```python
from build123d import *

# Parameters (mm, degrees)
BOSS_EXTRU_1_DEPTH      = 3.5
ENL_V_MAT_EXTRU_1_DEPTH = 0.2
ESQUISSE3_R             = 2.3
BOSS_EXTRU_2_DEPTH      = 1.3
CONG_1_R                = 0.1
CONG_2_R                = 0.01
ESQUISSE4_W             = 1.998545811
ESQUISSE4_H             = 1.004796591
BOSS_EXTRU_3_DEPTH      = 0.1
ESQUISSE5_W             = 2.001116517
ESQUISSE5_H             = 1.004085413
BOSS_EXTRU_4_DEPTH      = 0.1


with BuildPart() as part:
    # Esquisse1 → Boss.-Extru.1 (new body)
    with BuildSketch(Plane.XY):
        with BuildLine():
            Line((0.5, 0), (5.5, 0))
            ThreePointArc((5.5, 0), (5.853553391, 0.146446609), (6, 0.5))
            Line((6, 0.5), (6, 5.5))
            ThreePointArc((6, 5.5), (5.853553391, 5.853553391), (5.5, 6))
            Line((5.5, 6), (0.5, 6))
            ThreePointArc((0.5, 6), (0.146446609, 5.853553391), (0, 5.5))
            Line((0, 5.5), (0, 0.5))
            ThreePointArc((0, 0.5), (0.146446609, 0.146446609), (0.5, 0))
        make_face()
    extrude(amount=BOSS_EXTRU_1_DEPTH)

    # Esquisse2 → Enlèv. mat.-Extru.1 (cut)
    with BuildSketch(Plane.XY.offset(3.5)):
        with BuildLine():
            Line((1.11, 0.61), (4.89, 0.61))
            ThreePointArc((4.89, 0.61), (5.243553391, 0.756446609), (5.39, 1.11))
            Line((5.39, 1.11), (5.39, 4.89))
            ThreePointArc((5.39, 4.89), (5.243553391, 5.243553391), (4.89, 5.39))
            Line((4.89, 5.39), (1.11, 5.39))
            ThreePointArc((1.11, 5.39), (0.756446609, 5.243553391), (0.61, 4.89))
            Line((0.61, 4.89), (0.61, 1.11))
            ThreePointArc((0.61, 1.11), (0.756446609, 0.756446609), (1.11, 0.61))
        make_face()
    extrude(amount=-ENL_V_MAT_EXTRU_1_DEPTH, mode=Mode.SUBTRACT)

    # Esquisse3 → Boss.-Extru.2 (add)
    with BuildSketch(Plane.XY.offset(3.3)):
        with Locations((2.9955811, 3.011293081)):
            Circle(ESQUISSE3_R)
    extrude(amount=BOSS_EXTRU_2_DEPTH)

    # Congé1
    cong_1_edges = [part.edges().sort_by_distance(p)[0] for p in [
        (0.6955811, 3.011293081, 4.6),
    ]]
    fillet(cong_1_edges, radius=CONG_1_R)

    # Congé2
    cong_2_edges = [part.edges().sort_by_distance(p)[0] for p in [
        (5.243553391, 0.756446609, 3.3),
        (3, 0.61, 3.3),
        (0.756446609, 0.756446609, 3.3),
        (0.61, 3, 3.3),
        (0.756446609, 5.243553391, 3.3),
        (3, 5.39, 3.3),
        (5.243553391, 5.243553391, 3.3),
        (5.39, 3, 3.3),
        (5.243553391, 0.756446609, 3.5),
        (5.39, 3, 3.5),
        (5.243553391, 5.243553391, 3.5),
        (3, 5.39, 3.5),
        (0.756446609, 5.243553391, 3.5),
        (0.61, 3, 3.5),
        (0.756446609, 0.756446609, 3.5),
        (3, 0.61, 3.5),
    ]]
    fillet(cong_2_edges, radius=CONG_2_R)

    # Esquisse4 → Boss.-Extru.3 (add)
    with BuildSketch(Plane.XZ):
        with Locations((2.998734602, 0.502398296)):
            Rectangle(ESQUISSE4_W, ESQUISSE4_H)
    extrude(amount=BOSS_EXTRU_3_DEPTH)

    # Esquisse5 → Boss.-Extru.4 (add)
    with BuildSketch(Plane(origin=(0, 6, 0), x_dir=(1, 0, 0), z_dir=(0, 1, 0))):
        with Locations((2.997449249, -0.502042707)):
            Rectangle(ESQUISSE5_W, ESQUISSE5_H)
    extrude(amount=BOSS_EXTRU_4_DEPTH)


solid = part.part
```
Source: CAD feature listing. Evaluate the final solid. Frame: model axes, mm. A direction names the side the tool comes from. Coordinates: 2 decimals unless noted, no trailing zeros. Order: outer loops, then holes, each group sorted by start corner. A loop starts at its lowest first (then second) coordinate and runs counter-clockwise, first axis right, second up. Notation, with made-up numbers: (-27.75, 59) - (-1.75, 59) arc R21 cw to (-1.75, 95) - close; hole circle Ø8 at (77.5, 9). An arc over 180 degrees is marked (long way). One line per item, written item: value.
1) Cut plane A-A on z = 1.1. Output: boundary loops of the cut face in (x, y).
Computed values:
outline: (0, 0.5) arc R0.5 ccw to (0.5, 0) - (5.5, 0) arc R0.5 ccw to (6, 0.5) - (6, 5.5) arc R0.5 ccw to (5.5, 6) - (0.5, 6) arc R0.5 ccw to (0, 5.5) - close
2) Reachability of faces 1 (the face through (3, 3, 4.6)), 2 (the face through (2.497, 0.766, 3.892)) from +Z, -Z, +X, -X, +Y, -Y: full face, straight path, thin tool, end or side. Return the list, or none.
Computed values:
face 1: +Z, +X, -X, +Y, -Y
face 2: +Z
3) Ray query, line 1 (Y direction, x = 1.2, z = 3); line 2 (X direction, y = 3, z = 3.85); line 3 (Z direction, x = 0.55, y = 1.5). Return the intervals inside material, ascending. Write a range as [from, to].
Computed values:
line 1: y = [0, 6]
line 2: x = [0.7, 5.3]
line 3: z = [0, 3.5]
4) Contact query for a flat-ended pin moving along its axis: pin 1 (1 mm diameter, centred on x = 2.5, z = 2, fed in from +Y). Output: stop coordinate, or through.
Computed values:
pin 1: stops at y = 6
5) Cut plane B-B on z = 4.25. Output: boundary loops of the cut face in (x, y).
Computed values:
outline: circle Ø4.6 at (3, 3.01)
